from build123d import *

# Parameters (mm, degrees)
F0_W           = 67.1
F0_H           = 38.6
F1_DEPTH       = 5
F2_DEPTH       = 5
F3_D           = 2.2
F3_CSINK_D     = 6.72
F3_CSINK_ANGLE = 90
F5_D           = 2.2
F7_DEPTH       = 25
F8_R           = 5


with BuildPart() as f1:
    # F0 (on Top) → F1 (new body)
    with BuildSketch(Plane.XY):
        with BuildLine():
            ThreePointArc((40.55, 16.8), (39.231981, 19.981981), (36.05, 21.3))
            Line((36.05, 21.3), (-36.05, 21.3))
            ThreePointArc((-36.05, 21.3), (-39.231981, 19.981981), (-40.55, 16.8))
            Line((-40.55, 16.8), (-40.55, -16.8))
            ThreePointArc((-40.55, -16.8), (-39.231981, -19.981981), (-36.05, -21.3))
            Line((-36.05, -21.3), (-14.45, -21.3))
            Line((-14.45, -21.3), (36.05, -21.3))
            ThreePointArc((36.05, -21.3), (39.231981, -19.981981), (40.55, -16.8))
            Line((40.55, -16.8), (40.55, 16.8))
        make_face()
        Rectangle(F0_W, F0_H, mode=Mode.SUBTRACT)
    extrude(amount=F1_DEPTH)

    # F0 (on Top) → F2 (join)
    with BuildSketch(Plane.XY):
        with BuildLine():
            Line((-36.05, 21.3), (36.05, 21.3))
            ThreePointArc((36.05, 21.3), (39.231981, 19.981981), (40.55, 16.8))
            Line((40.55, 16.8), (42.55, 16.8))
            ThreePointArc((42.55, 16.8), (40.646194, 21.396194), (36.05, 23.3))
            Line((36.05, 23.3), (-36.05, 23.3))
            ThreePointArc((-36.05, 23.3), (-40.646194, 21.396194), (-42.55, 16.8))
            Line((-42.55, 16.8), (-42.55, -16.8))
            ThreePointArc((-42.55, -16.8), (-40.646194, -21.396194), (-36.05, -23.3))
            Line((-36.05, -23.3), (-14.45, -23.3))
            Line((-14.45, -23.3), (-14.45, -21.3))
            Line((-14.45, -21.3), (-36.05, -21.3))
            ThreePointArc((-36.05, -21.3), (-39.231981, -19.981981), (-40.55, -16.8))
            Line((-40.55, -16.8), (-40.55, 16.8))
            ThreePointArc((-40.55, 16.8), (-39.231981, 19.981981), (-36.05, 21.3))
        make_face()
        with BuildLine():
            Line((42.55, 16.8), (40.55, 16.8))
            Line((40.55, 16.8), (40.55, -16.8))
            ThreePointArc((40.55, -16.8), (39.231981, -19.981981), (36.05, -21.3))
            Line((36.05, -21.3), (-14.45, -21.3))
            Line((-14.45, -21.3), (-14.45, -23.3))
            Line((-14.45, -23.3), (36.05, -23.3))
            ThreePointArc((36.05, -23.3), (40.646194, -21.396194), (42.55, -16.8))
            Line((42.55, -16.8), (42.55, 16.8))
        make_face()
    extrude(amount=F2_DEPTH)

    # F3 (through all)
    with Locations(Plane(origin=(0, 0, 0), x_dir=(1, 0, 0), z_dir=(0, 0, -1))):
        with Locations((37.2, 14.05), (37.2, -14.05), (-37.2, -14.05), (-37.2, 14.05)):
            CounterSinkHole(F3_D / 2, F3_CSINK_D / 2, counter_sink_angle=F3_CSINK_ANGLE)

    # F5 (through all)
    with Locations(Plane.YZ.offset(42.55)):
        with Locations((0, 2.5)):
            Hole(F5_D / 2)

    # F6 (on face) → F7 (join)
    with BuildSketch(Plane.XY.offset(5)):
        with BuildLine():
            Line((-42.55, 16.8), (-42.55, -16.8))
            Line((-42.55, -16.8), (-40.55, -16.8))
            Line((-40.55, -16.8), (-40.55, 16.8))
            ThreePointArc((-40.55, 16.8), (-39.231981, 19.981981), (-36.05, 21.3))
            Line((-36.05, 21.3), (20.95, 21.3))
            Line((20.95, 21.3), (20.95, 23.3))
            Line((20.95, 23.3), (-36.05, 23.3))
            ThreePointArc((-36.05, 23.3), (-40.646194, 21.396194), (-42.55, 16.8))
        make_face()
    extrude(amount=F7_DEPTH)

    # F8
    f8_edges = [f1.edges().sort_by_distance(p)[0] for p in [
        (-41.55, -16.8, 30),
        (20.95, 22.3, 30),
        (20.95, 22.3, 5),
    ]]
    fillet(f8_edges, radius=F8_R)


solid = f1.part
Model file for the job. Use its own axes, mm. A direction names the side the tool comes from. Give positions to 0.01 mm unless a question says otherwise; leave off trailing zeros. Loops run counter-clockwise (first coordinate to the right, second up) from the corner with the lowest first, then second, coordinate; pieces in that order, holes last.
1) Saw through at D-D (x = -37.2). Write the cut outline in (y, z).
2) Wall check: line 1 (X direction, y = 14.05, z = 3.85); line 2 (Y direction, x = -4, z = 4.75); line 3 (Z direction, x = -36.25, y = 0). Give the ranges that are in metal, low to high.
3) Pull direction Y, two halves, no side cores. Call faces 4 (the flat face through (0, 19.3, 2)), 5 (the flat face through (-42.55, 0, 15)), 6 (the flat face through (-42, -16.8, 15)): +Y half, -Y half, draft (parallel to the pull), parting line (faces both ways), or undercut.
4) Flat gauge pins, fed straight in: pin 1 Ø12.5 at (y, z) = (-0.5, 18.5) entering from +X; pin 2 Ø3 at (x, y) = (-37.2, 14.05) entering from -Z; pin 3 Ø7.5 at (x, z) = (4, 21.5) entering from -Y. Where does each tip first touch, or does it go through?
5) Tool access for faces 1 (the flat face through (0, -19.3, 2)), 2 (the flat face through (20.95, 22, 17)), 3 (the cylindrical face through (-39.267, 19.947, 17.325)): list every direction of +Z, -Z, +X, -X, +Y, -Y with a clear straight run to the whole face (end or side of a thin tool).
6) Saw through at B-B (y = 14.05). Write the cut outline in (x, z).
7) Saw through at A-A (y = -2.5). Write the cut outline in (x, z), plus the area to 3 significant figures.
8) Saw through at C-C (x = -8.5). Write the cut outline in (y, z).
Answer block:
1. outline: (-23.2, 0) - (-17.41, 0) - (-15.15, 2.26) - (-15.15, 5) - (-23.2, 5) - close; (-12.95, 2.26) - (-10.69, 0) - (10.69, 0) - (12.95, 2.26) - (12.95, 5) - (-12.95, 5) - close; (15.15, 2.26) - (17.41, 0) - (23.2, 0) - (23.2, 30) - (21.15, 30) - (21.15, 5) - (15.15, 5) - close; hole circle Ø2.2 at (0, 2.5)
2. line 1: x = -42.55 to -38.3, -36.1 to -33.55, 33.55 to 36.1, 38.3 to 42.55
2. line 2: y = -23.3 to -19.3, 19.3 to 23.3
2. line 3: z = 0 to 1.4, 3.6 to 5
3. face 4: undercut
3. face 5: draft
3. face 6: -Y half
4. pin 1: stops at x = -40.55
4. pin 2: stops at z = 1.86
4. pin 3: stops at y = 21.3
5. face 1: +Z, -Z
5. face 2: +Z, +X, +Y, -Y
5. face 3: +Z, +X, -Y
6. outline: (-42.55, 0) - (-40.56, 0) - (-38.3, 2.26) - (-38.3, 5) - (-40.55, 5) - (-40.55, 30) - (-42.55, 30) - close; (-36.1, 2.26) - (-33.84, 0) - (-33.55, 0) - (-33.55, 5) - (-36.1, 5) - close; (33.55, 0) - (33.84, 0) - (36.1, 2.26) - (36.1, 5) - (33.55, 5) - close; (38.3, 2.26) - (40.56, 0) - (42.55, 0) - (42.55, 5) - (38.3, 5) - close
7. outline: (-42.55, 0) - (-33.55, 0) - (-33.55, 5) - (-40.55, 5) - (-40.55, 30) - (-42.55, 30) - close; (33.55, 0) - (42.55, 0) - (42.55, 5) - (33.55, 5) - close
7. area: 140 mm2
8. outline: (-23.3, 0) - (-19.3, 0) - (-19.3, 5) - (-23.3, 5) - close; (19.3, 0) - (23.3, 0) - (23.3, 30) - (21.3, 30) - (21.3, 5) - (19.3, 5) - close
